```python
from build123d import *

# Parameters (mm, degrees)
SKETCH1_R           = 15
BOSS_EXTRUDE1_DEPTH = 10
SKETCH2_R           = 10
CUT_EXTRUDE1_DEPTH  = 1


with BuildPart() as part:
    # Sketch1 → Boss-Extrude1 (new body)
    with BuildSketch(Plane(origin=(0, 0, 0), x_dir=(1, 0, 0), z_dir=(0, 1, 0))):
        Circle(SKETCH1_R)
    extrude(amount=BOSS_EXTRUDE1_DEPTH)

    # Sketch3 → Cut-Revolve1 (revolve, cut)
    with BuildSketch(Plane(origin=(0, 0, 0), x_dir=(-1, 0, 0), z_dir=(0, -1, 0))):
        with BuildLine():
            Line((0, 5), (0, -5))
            ThreePointArc((0, -5), (5, 0), (0, 5))
        make_face()
    revolve(axis=Axis((0, 0, -5), (0, 0, 1)), mode=Mode.SUBTRACT)

    # Sketch2 → Cut-Extrude1 (cut)
    with BuildSketch(Plane(origin=(0, 10, 0), x_dir=(1, 0, 0), z_dir=(0, 1, 0))):
        Circle(SKETCH2_R)
        with BuildLine():
            Line((-0.5, -0.499807062), (-0.5, -8.986100378))
            ThreePointArc((-0.5, -8.986100378), (-6.36402935, -6.363892711), (-8.986111111, -0.499807062))
            Line((-8.986111111, -0.499807062), (-0.5, -0.499807062))
        make_face(mode=Mode.SUBTRACT)
        with BuildLine():
            Line((0.499807062, 8.986111111), (0.499807062, 0.499807062))
            Line((0.499807062, 0.499807062), (8.986111111, 0.499807062))
            ThreePointArc((8.986111111, 0.499807062), (6.363961031, 6.363961031), (0.499807062, 8.986111111))
        make_face(mode=Mode.SUBTRACT)
        with BuildLine():
            Line((-0.5, 8.986100378), (-0.5, 0.499807062))
            Line((-0.5, 0.499807062), (-8.986111111, 0.499807062))
            ThreePointArc((-8.986111111, 0.499807062), (-6.36402935, 6.363892711), (-0.5, 8.986100378))
        make_face(mode=Mode.SUBTRACT)
        with BuildLine():
            Line((8.986111111, -0.499807062), (0.499807062, -0.499807062))
            Line((0.499807062, -0.499807062), (0.499807062, -8.986111111))
            ThreePointArc((0.499807062, -8.986111111), (6.363961031, -6.363961031), (8.986111111, -0.499807062))
        make_face(mode=Mode.SUBTRACT)
    extrude(amount=-CUT_EXTRUDE1_DEPTH, mode=Mode.SUBTRACT)


solid = part.part
```
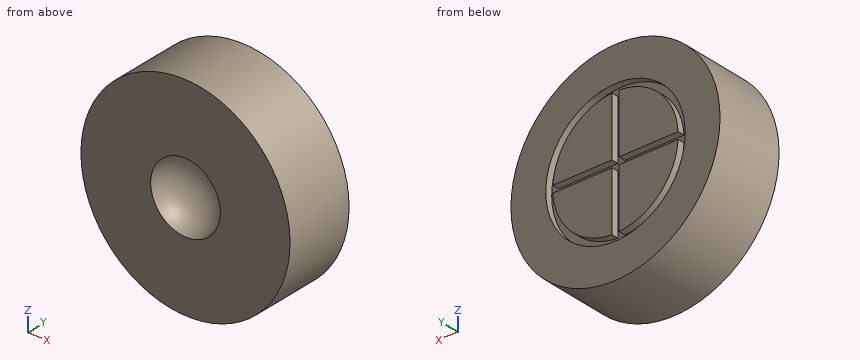
Can you work these out from the model? Positions are in its coordinate system, mm. Give positions to 0.01 mm unless a question says otherwise; leave off trailing zeros. Loops run counter-clockwise (first coordinate to the right, second up) from the corner with the lowest first, then second, coordinate; pieces in that order, holes last. Notation, with made-up numbers: M 62.25,79.25 L 104.25,79.25 A22 cw 104.25,108.25 Z; hole C 32,0.5 d10. An arc over 180 degrees is marked long. Use one line per item in the form item = value. Start each with the question number.
(1) I want a section at A-A, the plane x = 0. Write out the boundary of the cut face in (y, z).
(2) I want a section at B-B, the plane z = 0. Write out the boundary of the cut face in (x, y), and give its area (3 significant figures).
(3) I'm going to push flat-ended pins straight in: P1, Ø5, axis at x = 11.5, y = 6.5, coming from the -Z side; P2, Ø10, axis at x = -11.5, z = -11.5, coming from the -Y side; P3, Ø0.8, axis at y = 9.5, z = 3, coming from the +X side; P4, Ø0.5, axis at x = -6, y = 9.5, coming from the -Z side. Where does each tip first touch, or does it pass through?
(4) I want a section at D-D, the plane y = 1. Write out the boundary of the cut face in (x, z), and give its area (3 significant figures).
(5) Please list where these lines run through material, in increasing order: line 1 (Z direction, x = 0, y = 9.6); line 2 (Z direction, x = -1.5, y = 9.25).
(6) I want a section at C-C, the plane y = 7.75. Write out the boundary of the cut face in (x, z), and give its area (3 significant figures).
Worked out:
q1.outline = M 0,-15 L 10,-15 L 10,-10 L 9,-10 L 9,10 L 10,10 L 10,15 L 0,15 L 0,5 A5 cw 0,-5 Z
q2.outline = M -15,0 L -5,0 A5 cw 5,0 L 15,0 L 15,10 L 10,10 L 10,9 L -10,9 L -10,10 L -15,10 Z
q2.area = 241 mm²
q3.P1 = -12
q3.P2 = 0
q3.P3 = 14.77
q3.P4 = -13.85
q4.outline = C 0,0 d30; hole C 0,0 d9.8
q4.area = 631 mm²
q5.line_1 = -15 to -10, 10 to 15
q5.line_2 = -14.92 to -9.89, -8.87 to -0.5, 0.5 to 8.87, 9.89 to 14.92
q6.outline = C 0,0 d30
q6.area = 707 mm²
